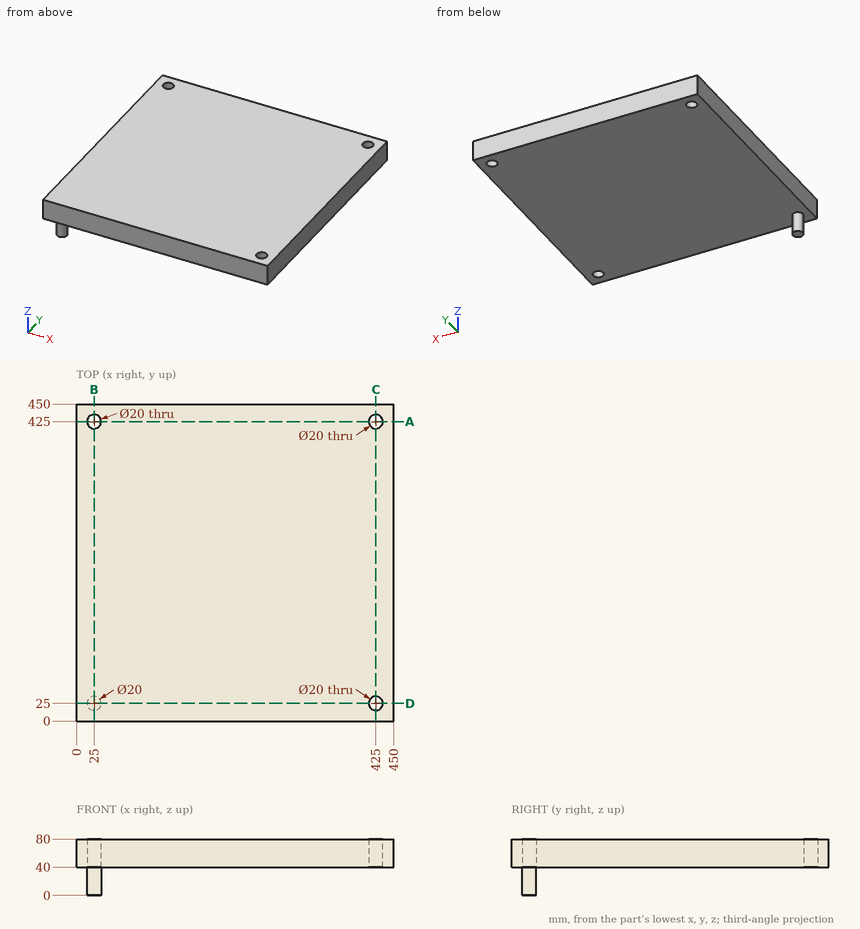
Verification items for this drawing (mm, ordinates from the low corner). Coordinates: 2 decimals unless noted, no trailing zeros. Order: outer loops, then holes, each group sorted by start corner. A loop starts at its lowest first (then second) coordinate and runs counter-clockwise, first axis right, second up. Notation, with made-up numbers: (41, -38) - (53, -38) arc R13 cw to (53, -27) - close; hole circle Ø2 at (29.5, 10). An arc over 180 degrees is marked (long way). Use one line per item in the form item = value.
1. Section check A-A (y = 425). Record the boundary of the cut face in (x, z).
Here are the results:
outline = (0, 40) - (15, 40) - (15, 80) - (0, 80) - close; (35, 40) - (415, 40) - (415, 80) - (35, 80) - close; (435, 40) - (450, 40) - (450, 80) - (435, 80) - close
2. Gauge pin test, flat ends, axial feed: pin 1 (12 mm diameter, centred on x = 54, y = 347.5, fed in from -Z); pin 2 (18 mm diameter, centred on x = 425, y = 425, fed in from -Z). Record the tip position at first contact, or that the pin passes through.
Here are the results:
pin_1 = 40
pin_2 = through
3. Scan lines: line 1 (X direction, y = 425, z = 66); line 2 (X direction, y = 25.5, z = 74). Record each from-to range of solid material in increasing order.
Here are the results:
line_1 = 0 to 15, 35 to 415, 435 to 450
line_2 = 0 to 415.01, 434.99 to 450
4. Section check B-B (x = 25). Record the boundary of the cut face in (y, z).
Here are the results:
outline = (0, 40) - (15, 40) - (15, 0) - (35, 0) - (35, 40) - (415, 40) - (415, 80) - (0, 80) - close; (435, 40) - (450, 40) - (450, 80) - (435, 80) - close
